Read the model definition and answer for the solid it produces. Units are mm, in the model's axes. Face numbers are marked on the shaded views. A direction names the side the tool comes from. Round coordinates to 2 decimals unless told otherwise and drop trailing zeros. Loops run counter-clockwise (first coordinate to the right, second up) from the corner with the lowest first, then second, coordinate; pieces in that order, holes last. Notation, with made-up numbers: M 0.5,-36.75 L 20.5,-36.75 A13 cw 20.5,-14.75 Z; hole C 22,-38 d7. An arc over 180 degrees is marked long. Write each question's results on one line, items separated by ' | '.
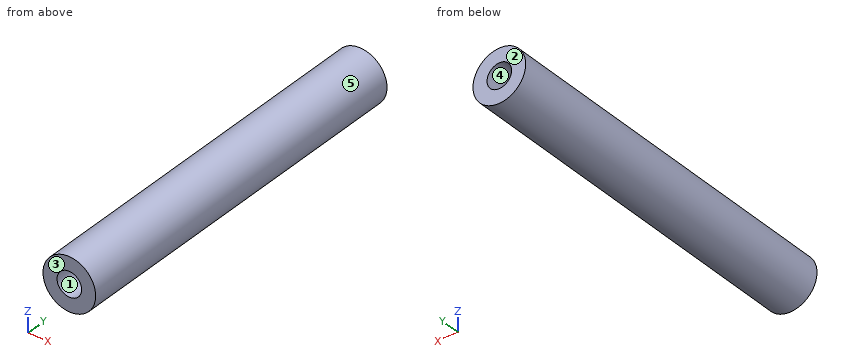
```python
from build123d import *

# Parameters (mm, degrees)
SKETCH1_R           = 3
SKETCH1_R_2         = 1.4
BOSS_EXTRUDE1_DEPTH = 42
BOSS_EXTRUDE2_START = 10
SKETCH1_3_R         = 1.4
BOSS_EXTRUDE2_DEPTH = 22


with BuildPart() as part:
    # Sketch1 → Boss-Extrude1 (new body)
    with BuildSketch(Plane(origin=(0, 0, 0), x_dir=(1, 0, 0), z_dir=(0, 1, 0))):
        with Locations(Location((0, 0, 0), (0, 0, 90))):
            Circle(SKETCH1_R)
        with Locations(Location((0, 0, 0), (0, 0, 90))):
            Circle(SKETCH1_R_2, mode=Mode.SUBTRACT)
    extrude(amount=BOSS_EXTRUDE1_DEPTH)

    # Sketch1_3 → Boss-Extrude2 (add)
    with BuildSketch(Plane(origin=(0, 0, 0), x_dir=(1, 0, 0), z_dir=(0, 1, 0)).offset(BOSS_EXTRUDE2_START)):
        with Locations(Location((0, 0, 0), (0, 0, 90))):
            Circle(SKETCH1_3_R)
    extrude(amount=BOSS_EXTRUDE2_DEPTH)


solid = part.part
```
1. Find section A-A, the plane x = 0. Give the vertices of the cut face in (y, z).
Completed:
outline: M 0,-3 L 42,-3 L 42,-1.4 L 32,-1.4 L 32,1.4 L 42,1.4 L 42,3 L 0,3 L 0,1.4 L 10,1.4 L 10,-1.4 L 0,-1.4 Z
2. Which of the six approach directions +Z, -Z, +X, -X, +Y, -Y give full straight-line access (tool end or side, diameter ignored) to the marked faces 1 and 2?
Completed:
face 1: -Y | face 2: +Z, -Z, +X, -X, +Y
3. Find section D-D, the plane y = 15.5. Give the vertices of the cut face in (x, z), then the cut area to 3 significant figures.
Completed:
outline: C 0,0 d6 | area: 28.3 mm2
4. Find section B-B, the plane z = 0. Give the vertices of the cut face in (x, y), then the cut area to 3 significant figures.
Completed:
outline: M -3,0 L -1.4,0 L -1.4,10 L 1.4,10 L 1.4,0 L 3,0 L 3,42 L 1.4,42 L 1.4,32 L -1.4,32 L -1.4,42 L -3,42 Z | area: 196 mm2
5. Given P1, Ø2, axis at x = 0, z = 0, coming from the +Y side, flat-ended and moving along its own axis, determine where the tip first touches the part or whether it passes through.
Completed:
P1: stops at y = 32
6. Find the intervals of material crossed by L1, parallel to X at y = 6, z = 0; L2, parallel to Y at x = -0.2, z = -0.3; L3, parallel to Z at x = -0.95, y = 16, in increasing order.
Completed:
L1: x = -3 to -1.4, 1.4 to 3 | L2: y = 10 to 32 | L3: z = -2.85 to 2.85
7. Determine the mould class of the marked faces 3, 4 and 5 for opening direction X: released by +X, released by -X, zero draft, split by the parting line, or undercut.
Completed:
face 3: zero draft | face 4: undercut | face 5: split by the parting line
8. Find section C-C, the plane y = 36. Give the vertices of the cut face in (x, z).
Completed:
outline: C 0,0 d6; hole C 0,0 d2.8
